Source: CAD feature listing. Evaluate the final solid. Frame: model axes, mm. A direction names the side the tool comes from. Coordinates: 2 decimals unless noted, no trailing zeros. Order: outer loops, then holes, each group sorted by start corner. A loop starts at its lowest first (then second) coordinate and runs counter-clockwise, first axis right, second up.
```python
from build123d import *

# Parameters (mm, degrees)
F0_W     = 151.572406292
F0_H     = 153.1009078026
F1_DEPTH = 6.35
F2_SIZE  = 5.08
F3_SIZE  = 5.08
F4_SIZE  = 5.08
F5_SIZE  = 5.08
F6_W     = 17.9464835674
F6_H     = 13.5393217206
F7_DEPTH = 0.762
F8_W     = 21.0372619331
F8_H     = 13.5393217206
F9_DEPTH = 0.762
F10_SIZE = 5.08
F11_SIZE = 5.08
F12_SIZE = 5.08
F13_SIZE = 5.08


with BuildPart() as f1:
    # F0 (on Top) → F1 (new body, symmetric)
    with BuildSketch(Plane.XY):
        with Locations((-0.1000165939, 0.1238584518)):
            Rectangle(F0_W, F0_H)
    extrude(amount=F1_DEPTH, both=True)

    # F2
    f2_edges = [f1.edges().sort_by_distance(p)[0] for p in [
        (-0.100017, -76.426595, 6.35),
    ]]
    chamfer(f2_edges, length=F2_SIZE)

    # F3
    f3_edges = [f1.edges().sort_by_distance(p)[0] for p in [
        (-0.100017, 76.674312, 6.35),
    ]]
    chamfer(f3_edges, length=F3_SIZE)

    # F4
    f4_edges = [f1.edges().sort_by_distance(p)[0] for p in [
        (75.686187, 0.123858, 6.35),
    ]]
    chamfer(f4_edges, length=F4_SIZE)

    # F5
    f5_edges = [f1.edges().sort_by_distance(p)[0] for p in [
        (-75.88622, 0.123858, 6.35),
    ]]
    chamfer(f5_edges, length=F5_SIZE)

    # F6 (on face) → F7 (cut)
    with BuildSketch(Plane(origin=(0, 0, -6.35), x_dir=(1, 0, 0), z_dir=(0, 0, -1))):
        with Locations((32.9451402649, -69.9046514928)):
            Rectangle(F6_W, F6_H)
    extrude(amount=-F7_DEPTH, mode=Mode.SUBTRACT)

    # F8 (on face) → F9 (cut)
    with BuildSketch(Plane(origin=(0, 0, -6.35), x_dir=(1, 0, 0), z_dir=(0, 0, -1))):
        with Locations((-35.0907575339, -69.9046514928)):
            Rectangle(F8_W, F8_H)
    extrude(amount=-F9_DEPTH, mode=Mode.SUBTRACT)

    # F10
    f10_edges = [f1.edges().sort_by_distance(p)[0] for p in [
        (75.686187, -76.426595, -2.54),
    ]]
    chamfer(f10_edges, length=F10_SIZE)

    # F11
    f11_edges = [f1.edges().sort_by_distance(p)[0] for p in [
        (75.686187, 76.674312, -2.54),
    ]]
    chamfer(f11_edges, length=F11_SIZE)

    # F12
    f12_edges = [f1.edges().sort_by_distance(p)[0] for p in [
        (-75.88622, 76.674312, -2.54),
    ]]
    chamfer(f12_edges, length=F12_SIZE)

    # F13
    f13_edges = [f1.edges().sort_by_distance(p)[0] for p in [
        (-75.88622, -76.426595, -2.54),
    ]]
    chamfer(f13_edges, length=F13_SIZE)


solid = f1.part
```
Q1. Pin query (flat end, axial travel): P1, Ø0.8, axis at y = 72.5, z = -6, coming from the +X side; P2, Ø4, axis at x = 36, y = 73, coming from the -Z side. Return the tip coordinate at first contact, or that it passes through.
Solutions:
P1: stops at x = 75.18
P2: stops at z = -5.59
Q2. Material intervals for line 1 along X through (y, z) = (-32, 3.5); line 2 along Y through (x, z) = (40.5, 3.75); line 3 along Y through (x, z) = (-54, 4.75), sorted ascending.
Solutions:
line 1: x = -73.66 to 73.46
line 2: y = -73.95 to 74.19
line 3: y = -72.95 to 73.19
Q3. Pull-direction query (X, two-part tool) for faces 3 (the flat face through (-75.886, -1, -2)), 4 (the flat face through (33, 70, -5.588)), 5 (the flat face through (-1.125, -73.922, 3.774)), 6 (the flat face through (73.182, -0.912, 3.774)); classes: pulls with the +X half, pulls with the -X half, needs draft (parallel to the pull), parting line crosses it, or undercut.
Solutions:
face 3: pulls with the -X half
face 4: undercut
face 5: needs draft
face 6: pulls with the +X half
Q4. Set-up query: faces 1 (the flat face through (-1, 1, 6.35)), 2 (the flat face through (-35, 70, -5.588)). Return all of +Z, -Z, +X, -X, +Y, -Y with unobstructed straight access to the full face (end or side cutting, diameter ignored); none if empty.
Solutions:
face 1: +Z, +X, -X, +Y, -Y
face 2: -Z, +Y
Q5. Section query A-A on x = -37.5. Output: boundary loops of the cut face in (y, z) (3 decimals), plus the area to 3 significant figures.
Solutions:
outline: (-76.427, -6.35) - (63.135, -6.35) - (63.135, -5.588) - (76.674, -5.588) - (76.674, 1.27) - (71.594, 6.35) - (-71.347, 6.35) - (-76.427, 1.27) - close
area: 1,910 mm2
